Design review of the part built by this model. Coordinates are the model's own, in mm. Coordinates: 2 decimals unless noted, no trailing zeros. Order: outer loops, then holes, each group sorted by start corner. A loop starts at its lowest first (then second) coordinate and runs counter-clockwise, first axis right, second up. Notation, with made-up numbers: M 80.5,57 L 117.5,57 A17 ccw 117.5,69 Z; hole C -21,22.25 d9. An arc over 180 degrees is marked long. Answer in a Markdown table with one row per item.
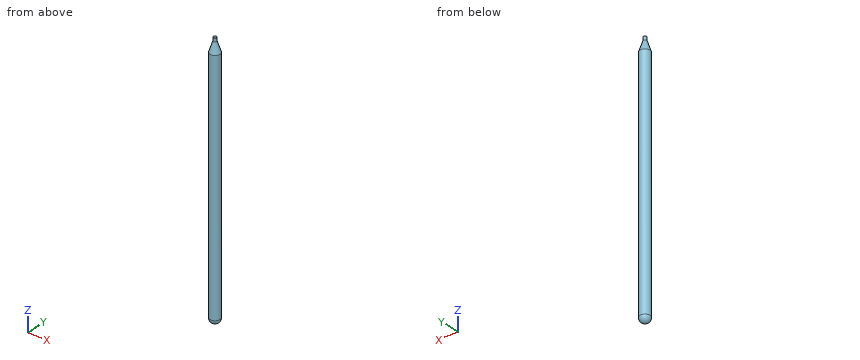
from build123d import *

# Parameters (mm, degrees)
CROQUIS3_R              = 3
SALIENTE_EXTRUIR2_DEPTH = 144
REDONDEO2_R             = 3
CROQUIS6_R              = 1
SALIENTE_EXTRUIR3_DEPTH = 2


with BuildPart() as part:
    # Croquis3 → Saliente-Extruir2 (new body)
    with BuildSketch(Plane.XY):
        Circle(CROQUIS3_R)
    extrude(amount=SALIENTE_EXTRUIR2_DEPTH)

    # Redondeo2
    redondeo2_edges = [part.edges().sort_by_distance(p)[0] for p in [
        (-3, 0, 0),
    ]]
    fillet(redondeo2_edges, radius=REDONDEO2_R)

    # Recubrir2: read off the stored shape, not the designer's step
    # Recubrir2: loft between two sections, ruled curve by curve
    recubrir2_from = [
        Edge.make_bspline([(-0.049268062, 0.998785592, 150), (1.948303122, 1.097321715, 150), (2.046839245, -0.900249468, 150), (0.049268062, -0.998785592, 150), (-1.948303122, -1.097321715, 150), (-2.046839245, 0.900249468, 150), (-0.049268062, 0.998785592, 150)], [0, 0, 0, 0, 0.5, 0.5, 0.5, 1, 1, 1, 1], 3, [1, 0.333333333, 0.333333333, 1, 0.333333333, 0.333333333, 1]),
    ]
    recubrir2_to = [
        Edge.make_bspline([(-1.18105567, 2.757735938, 144), (4.334416207, 5.119847278, 144), (6.696527546, -0.395624599, 144), (1.18105567, -2.757735938, 144), (-4.334416207, -5.119847278, 144), (-6.696527546, 0.395624599, 144), (-1.18105567, 2.757735938, 144)], [0, 0, 0, 0, 0.5, 0.5, 0.5, 1, 1, 1, 1], 3, [1, 0.333333333, 0.333333333, 1, 0.333333333, 0.333333333, 1]),
    ]
    recubrir2 = Solid(Shell([*[Face.make_surface_from_curves(recubrir2_from[k], recubrir2_to[k]) for k in range(1)], Face(Wire(recubrir2_from)), Face(Wire(recubrir2_to))]))
    add(recubrir2)

    # Croquis6 → Saliente-Extruir3 (add)
    with BuildSketch(Plane.XY.offset(150)):
        with Locations(Location((0, 0, 0), (0, 0, 92.823995247))):
            Circle(CROQUIS6_R)
    extrude(amount=SALIENTE_EXTRUIR3_DEPTH)


solid = part.part
(1) Add section A-A, the plane z = 42. Give the boundary of the cut face in (x, y), and give its area (3 significant figures).
Return value:
| item | result |
|---|---|
| outline | C 0,0 d6 |
| area | 28.3 mm2 |
(2) For line 1 along Y through (x, z) = (0.25, 59.5); line 2 along Y through (x, z) = (2, 25.5), list the stretches that pass through material, from the lowest coordinate up. Write a range as from..to.
Return value:
| item | result |
|---|---|
| line 1 | y = -2.99..2.99 |
| line 2 | y = -2.24..2.24 |
(3) Insertion check: pin 1 Ø2 at (x, z) = (-2, 21.5) entering from -Y. The pin has a flat end and moves straight along its axis. Give the tip position at first contact, or say it passes through.
Return value:
| item | result |
|---|---|
| pin 1 | stops at y = -2.83 |
